Read the model definition and answer for the solid it produces. Units are mm, in the model's axes. A direction names the side the tool comes from. Give positions to 0.01 mm unless a question says otherwise; leave off trailing zeros. Order: outer loops, then holes, each group sorted by start corner. A loop starts at its lowest first (then second) coordinate and runs counter-clockwise, first axis right, second up. Notation, with made-up numbers: (-24, 45) - (16, 45) arc R15 cw to (16, 62) - close; hole circle Ø9 at (52, 50). An arc over 180 degrees is marked (long way). Return JSON: item names as keys, results as strings.
```python
from build123d import *

# Parameters (mm, degrees)
SKETCH2_W           = 50.8
SKETCH2_H           = 101.6
BOSS_EXTRUDE1_DEPTH = 50.8
SKETCH3_W           = 50.8
SKETCH3_H           = 76.2
BOSS_EXTRUDE2_DEPTH = 50.8
BOSS_EXTRUDE3_REACH = 138.783
SKETCH4_R           = 38.1
CHAMFER2_SIZE       = 25.4
HOLE1_D             = 50.8


with BuildPart() as part:
    # Sketch2 → Boss-Extrude1 (new, symmetric)
    with BuildSketch(Plane.XY):
        Rectangle(SKETCH2_W, SKETCH2_H)
    extrude(amount=BOSS_EXTRUDE1_DEPTH, both=True)

    # Sketch3 → Boss-Extrude2 (add)
    with BuildSketch(Plane(origin=(76.2, 0, 0), x_dir=(0, 0, -1), z_dir=(1, 0, 0))):
        with Locations((0, -12.7)):
            Rectangle(SKETCH3_W, SKETCH3_H)
    extrude(amount=-BOSS_EXTRUDE2_DEPTH)

    # Boss-Extrude3: up to this face of the body (flat: up to its plane)
    boss_extrude3_end = Plane(part.part.faces().sort_by_distance((0, 0, -50.8))[0])
    # Sketch4 → Boss-Extrude3 (add, up to the picked face)
    with BuildSketch(Plane.XY.offset(50.8), mode=Mode.PRIVATE) as boss_extrude3_sk1:
        with Locations((76.2, -12.7)):
            Circle(SKETCH4_R)
    boss_extrude3_tool1 = split(extrude(boss_extrude3_sk1.sketch, amount=-BOSS_EXTRUDE3_REACH, mode=Mode.PRIVATE), bisect_by=boss_extrude3_end, keep=Keep.BOTH, mode=Mode.PRIVATE)
    add(boss_extrude3_tool1.solids().sort_by(Axis((76.2, -12.7, 50.8), (0, 0, -1)))[0])

    # Chamfer2
    chamfer2_edges = [part.edges().sort_by_distance(p)[0] for p in [
        (0, 50.8, -50.8),
        (0, 50.8, 50.8),
    ]]
    chamfer(chamfer2_edges, length=CHAMFER2_SIZE)

    # Hole1 (through all)
    with Locations(Plane(origin=(76.2, -12.7, 50.8), x_dir=(1, 0, 0), z_dir=(0, 0, 1))):
        with Locations((0, 0)):
            Hole(HOLE1_D / 2)


solid = part.part
```
Q1. A cutting plane is placed at D-D (z = 11). Write down the section's boundary in (x, y).
Values:
{"outline": "(-25.4, -50.8) - (76.2, -50.8) arc R38.1 ccw to (76.2, 25.4) - (25.4, 25.4) - (25.4, 50.8) - (-25.4, 50.8) - close; hole circle Ø50.8 at (76.2, -12.7)"}
Q2. A cutting plane is placed at C-C (x = 60). Write down the section's boundary in (y, z), and give its area (3 significant figures).
Values:
{"outline": "(-50.8, -25.4) - (-47.18, -25.4) - (-47.18, -50.8) - (-32.26, -50.8) - (-32.26, 50.8) - (-47.18, 50.8) - (-47.18, 25.4) - (-50.8, 25.4) - close; (6.86, -50.8) - (21.78, -50.8) - (21.78, -25.4) - (25.4, -25.4) - (25.4, 25.4) - (21.78, 25.4) - (21.78, 50.8) - (6.86, 50.8) - close", "area": "3,400 mm²"}
Q3. Consider L1, parallel to X at y = -12, z = -34; L2, parallel to Y at x = 76, z = 7; L3, parallel to X at y = -12, z = -13. Determine where each line is inside the solid, lowest interval first.
Values:
{"L1": "x = -25.4 to 25.4, 38.11 to 50.81, 101.59 to 114.29", "L2": "y = -50.8 to -38.1, 12.7 to 25.4", "L3": "x = -25.4 to 50.81, 101.59 to 114.29"}
Q4. For faces 4 (the flat face through (34, -13, -25.4)), 5 (the flat face through (34, -13, 25.4)), 6 (the cylindrical face through (112.54, -1.26, 0.71)), determine the directions among +Z, -Z, +X, -X, +Y, -Y from which every point of the face is accessible in a straight line to the end or side of a thin tool.
Values:
{"face 4": "-Z", "face 5": "+Z", "face 6": "none"}
Q5. Given pin 1 (12 mm diameter, centred on x = 35, z = 18, fed in from +Y); pin 2 (4 mm diameter, centred on x = 1, z = -32.5, fed in from +Y); pin 3 (1.5 mm diameter, centred on x = 80.5, z = 23, fed in from -Y), each flat-ended and moving along its own axis, determine where each tip first touches the part or whether it passes through.
Values:
{"pin 1": "stops at y = 25.4", "pin 2": "stops at y = 45.7", "pin 3": "stops at y = -50.63"}
Q6. A cutting plane is placed at A-A (z = 39). Write down the section's boundary in (x, y).
Values:
{"outline": "(-25.4, -50.8) - (25.4, -50.8) - (25.4, 37.2) - (-25.4, 37.2) - close; circle Ø76.2 at (76.2, -12.7); hole circle Ø50.8 at (76.2, -12.7)"}
Q7. A cutting plane is placed at B-B (y = -12.7). Write down the section's boundary in (x, z), and give its area (3 significant figures).
Values:
{"outline": "(-25.4, -50.8) - (25.4, -50.8) - (25.4, -25.4) - (38.1, -25.4) - (38.1, -50.8) - (50.8, -50.8) - (50.8, 50.8) - (38.1, 50.8) - (38.1, 25.4) - (25.4, 25.4) - (25.4, 50.8) - (-25.4, 50.8) - close; (101.6, -50.8) - (114.3, -50.8) - (114.3, 50.8) - (101.6, 50.8) - close", "area": "8,390 mm²"}
Q8. Determine the mould class of faces 1 (the flat face through (25.4, 33, 1)), 2 (the flat face through (-25.4, -1, 1)), 3 (the flat face through (51, 25.4, 0)) for opening direction X: released by +X, released by -X, zero draft, split by the parting line, or undercut.
Values:
{"face 1": "undercut", "face 2": "released by -X", "face 3": "zero draft"}
